from build123d import *

# Parameters (mm, degrees)
SKETCH1_W           = 69.03
SKETCH1_H           = 54.27
BOSS_EXTRUDE1_DEPTH = 1.65
SKETCH2_R           = 2
BOSS_EXTRUDE2_DEPTH = 1.5
SKETCH3_W           = 4.44
SKETCH3_H           = 3.21
BOSS_EXTRUDE3_DEPTH = 2.44
SKETCH4_W           = 17.82
SKETCH4_H           = 44.88
BOSS_EXTRUDE4_DEPTH = 20


with BuildPart() as part:
    # Sketch1 → Boss-Extrude1 (new body)
    with BuildSketch(Plane(origin=(0, 0, 0), x_dir=(1, 0, 0), z_dir=(0, 1, 0))):
        Rectangle(SKETCH1_W, SKETCH1_H)
    extrude(amount=BOSS_EXTRUDE1_DEPTH)

    # Sketch2 → Boss-Extrude2 (add)
    with BuildSketch(Plane(origin=(0, 1.65, 0), x_dir=(1, 0, 0), z_dir=(0, 1, 0))):
        with Locations(Location((-16.095, -14.385, 0), (0, 0, 90))):
            Circle(SKETCH2_R)
        with Locations(Location((-16.095, -6.385, 0), (0, 0, 90))):
            Circle(SKETCH2_R)
    extrude(amount=BOSS_EXTRUDE2_DEPTH)

    # Sketch3 → Boss-Extrude3 (add)
    with BuildSketch(Plane(origin=(0, 1.65, 0), x_dir=(1, 0, 0), z_dir=(0, 1, 0))):
        with Locations((-25.195, -13.135)):
            Rectangle(SKETCH3_W, SKETCH3_H)
        with Locations((-25.195, -5.135)):
            Rectangle(SKETCH3_W, SKETCH3_H)
    extrude(amount=BOSS_EXTRUDE3_DEPTH)

    # Sketch4 → Boss-Extrude4 (add)
    with BuildSketch(Plane(origin=(0, 1.65, 0), x_dir=(1, 0, 0), z_dir=(0, 1, 0))):
        with Locations((6.925, 2.335)):
            Rectangle(SKETCH4_W, SKETCH4_H)
    extrude(amount=BOSS_EXTRUDE4_DEPTH)


solid = part.part
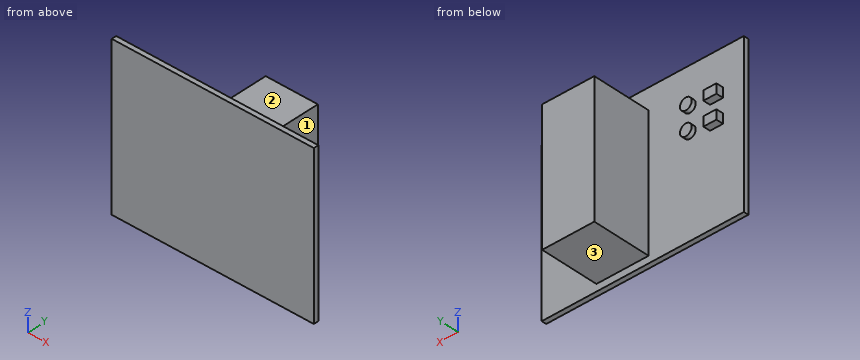
The listing builds one solid part. Answer for the finished solid, in the listing's coordinates (mm). Face numbers are marked on the shaded views. A direction names the side the tool comes from. Give positions to 0.01 mm unless a question says otherwise; leave off trailing zeros. Loops run counter-clockwise (first coordinate to the right, second up) from the corner with the lowest first, then second, coordinate; pieces in that order, holes last. Notation, with made-up numbers: (51, -7.75) - (56, -7.75) arc R6 cw to (56, -0.75) - close; hole circle Ø4 at (5.25, 33). An arc over 180 degrees is marked (long way). Write each question's results on one line, items separated by ' | '.
1. Find section A-A, the plane x = 9. Write down the section's boundary in (y, z) (3 decimals).
Resolved:
outline: (0, -27.135) - (1.65, -27.135) - (1.65, -24.775) - (21.65, -24.775) - (21.65, 20.105) - (1.65, 20.105) - (1.65, 27.135) - (0, 27.135) - close
2. Find section C-C, the plane y = 11.75. Write down the section's boundary in (x, z) (3 decimals).
Resolved:
outline: (-1.985, -24.775) - (15.835, -24.775) - (15.835, 20.105) - (-1.985, 20.105) - close
3. Flat-ended cylindrical pins translate along their axes: P1, Ø12, axis at x = -18.5, z = 21.5, coming from the -Y side; P2, Ø9, axis at x = 6, y = 9, coming from the +Z side (3 decimals); P3, Ø3, axis at x = 12.5, y = 9.5, coming from the -Z side (3 decimals); P4, Ø1.2, axis at x = -25.5, y = 3, coming from the +Z side. Find the tip coordinate at first contact, or state that the pin passes through.
Resolved:
P1: stops at y = 0 | P2: stops at z = 20.105 | P3: stops at z = -24.775 | P4: stops at z = 14.74
4. Which of the six approach directions +Z, -Z, +X, -X, +Y, -Y give full straight-line access (tool end or side, diameter ignored) to the marked faces 1, 2 and 3?
Resolved:
face 1: +Z, -Z, +X, +Y | face 2: +Z, +X, -X, +Y | face 3: -Z, +X, -X, +Y
5. Find section B-B, the plane z = 18.5. Write down the section's boundary in (x, y) (3 decimals), then the cut area to 3 significant figures.
Resolved:
outline: (-34.515, 0) - (34.515, 0) - (34.515, 1.65) - (15.835, 1.65) - (15.835, 21.65) - (-1.985, 21.65) - (-1.985, 1.65) - (-34.515, 1.65) - close | area: 470 mm^2
6. Find section D-D, the plane x = -20. Write down the section's boundary in (y, z) (3 decimals).
Resolved:
outline: (0, -27.135) - (1.65, -27.135) - (1.65, 27.135) - (0, 27.135) - close
7. Consider probe 1 along Y at (x, z) = (18, -8); probe 2 along X at (y, z) = (10, -12.5) (3 decimals); probe 3 along Z at (x, y) = (2, 17) (3 decimals). Determine where each line is inside the solid, lowest interval first. Write a range as from..to.
Resolved:
probe 1: y = 0..1.65 | probe 2: x = -1.985..15.835 | probe 3: z = -24.775..20.105
